Read the model definition and answer for the solid it produces. Units are mm, in the model's axes. Face numbers are marked on the shaded views. A direction names the side the tool comes from. Coordinates: 2 decimals unless noted, no trailing zeros. Loops run counter-clockwise (first coordinate to the right, second up) from the corner with the lowest first, then second, coordinate; pieces in that order, holes last. Notation, with made-up numbers: (-21, 50.25) -> (13, 50.25) arc R19 ccw to (13, 63.25) -> close; hole circle Ø7 at (-9, -23.5). An arc over 180 degrees is marked (long way). Answer as a JSON object with one key per item and string values. Group by question number.
Q1. Determine the mould class of the marked faces 5 and 6 for opening direction Y: released by +Y, released by -Y, zero draft, split by the parting line, or undercut.
Q2. Straight lines are drawn through the part: line 1 along Z through (x, y) = (0, -22); line 2 along Y through (x, z) = (-10.5, 36); line 3 along X through (y, z) = (-104, 100). For each, find the intervals that lie inside material, in ascending order. Write a range as [from, to].
Q3. The part is cut by section A-A on y = -67.5. Write down the section's boundary in (x, z).
Q4. For the marked faces 1, 2, 3 and 4, determine the directions among +Z, -Z, +X, -X, +Y, -Y from which every point of the face is accessible in a straight line to the end or side of a thin tool.
Q5. The part is cut by section C-C on y = -88.5. Write down the section's boundary in (x, z), and give its area (3 significant figures).
Q6. Each of these flat-tipped pins is pushed along its axis until it touches: P1, Ø12, axis at x = 15.5, z = 58, coming from the -Y side; P2, Ø16, axis at x = 0, z = 100, coming from the +Y side; P3, Ø4, axis at y = -67.5, z = 117, coming from the -X side. Where does it stop, or does it pass through?
from build123d import *

# Parameters (mm, degrees)
F4_R      = 15
F4_R_2    = 13.55
F6_DEPTH  = 150
F5_R      = 12
F5_R_2    = 10
F10_DEPTH = 4
F11_START = -12
F5_R_3    = 20
F11_DEPTH = 3


with BuildPart() as f6:
    # F4 (on Top) → F6 (new body, through all)
    with BuildSketch(Plane.XY):
        with Locations((0, -67.5)):
            Circle(F4_R)
        with Locations((0, -67.5)):
            Circle(F4_R_2, mode=Mode.SUBTRACT)
    extrude(amount=F6_DEPTH)

    # F5 (on offset) → F7 (join, up to the next surface of F6)
    with BuildSketch(Plane.XZ.offset(135)):
        with Locations((0, 100)):
            Circle(F5_R)
        with Locations((0, 100)):
            Circle(F5_R_2, mode=Mode.SUBTRACT)
        with Locations((0, 20)):
            Circle(F5_R)
        with Locations((0, 20)):
            Circle(F5_R_2, mode=Mode.SUBTRACT)
    extrude(until=Until.NEXT, dir=(0, 1, 0))

    # F9 (on plane+point) → F10 (cut)
    with BuildSketch(Plane.YZ.offset(15)):
        with BuildLine():
            ThreePointArc((-69.5, 119.5617376915), (-67.5, 120.25), (-65.5, 119.5617376915))
            Line((-65.5, 119.5617376915), (-65.5, 150))
            Line((-65.5, 150), (-69.5, 150))
            Line((-69.5, 150), (-69.5, 119.5617376915))
        make_face()
        with BuildLine():
            ThreePointArc((-69.5, 119.5617376915), (-68.9252192814, 114.0791696386), (-64.25, 117))
            ThreePointArc((-64.25, 117), (-64.5791696386, 118.4252192814), (-65.5, 119.5617376915))
            Line((-65.5, 119.5617376915), (-65.5, 117))
            Line((-65.5, 117), (-69.5, 117))
            Line((-69.5, 117), (-69.5, 119.5617376915))
        make_face()
        with BuildLine():
            Line((-65.5, 117), (-65.5, 119.5617376915))
            ThreePointArc((-65.5, 119.5617376915), (-67.5, 120.25), (-69.5, 119.5617376915))
            Line((-69.5, 119.5617376915), (-69.5, 117))
            Line((-69.5, 117), (-65.5, 117))
        make_face()
    extrude(amount=-F10_DEPTH, mode=Mode.SUBTRACT)

    # F5 (on offset) → F11 (join)
    with BuildSketch(Plane.XZ.offset(135).offset(F11_START)):
        with Locations((0, 100)):
            Circle(F5_R_3)
        with Locations((0, 100)):
            Circle(F5_R, mode=Mode.SUBTRACT)
        with Locations((0, 20)):
            Circle(F5_R_3)
        with Locations((0, 20)):
            Circle(F5_R, mode=Mode.SUBTRACT)
    extrude(amount=-F11_DEPTH)

    # F12: F6 across plane


with BuildPart() as f6_1:
    add(f6.part)
    add(f6.part.mirror(Plane.XZ.offset(67.5)))


solid = f6_1.part
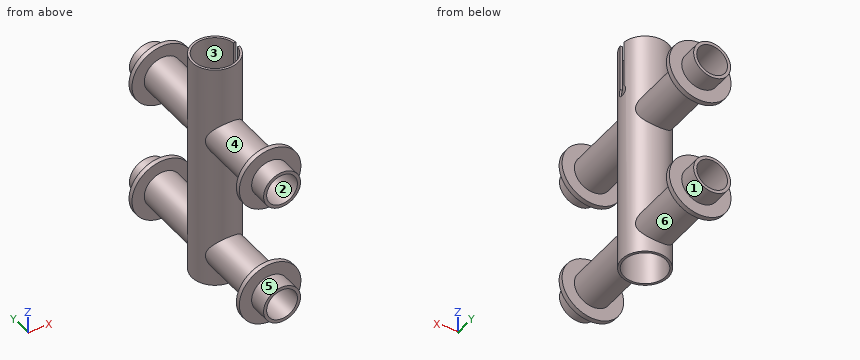
Final values:
{
 "1": {"face 5": "zero draft", "face 6": "undercut"},
 "2": {"line 1": "z = [8, 10], [30, 32], [88, 90], [110, 112]", "line 2": "y = [-123, -120], [-78.21, -76.06], [-58.94, -56.79], [-15, -12]", "line 3": "x = [-12, -10], [10, 12]"},
 "3": {"outline": "(-15, 0) -> (-13.55, 0) -> (-13.55, 150) -> (-15, 150) -> close; (13.55, 0) -> (15, 0) -> (15, 113.75) -> (13.55, 113.75) -> close"},
 "4": {"face 1": "+Y", "face 2": "-Y", "face 3": "+Z, -Z", "face 4": "none"},
 "5": {"outline": "circle Ø24 at (0, 20); circle Ø24 at (0, 100); hole circle Ø20 at (0, 20); hole circle Ø20 at (0, 100)", "area": "276 mm2"},
 "6": {"P1": "stops at y = -79.11", "P2": "stops at y = -52.5", "P3": "stops at x = -15"}
}
